Design review of the part built by this model. Coordinates are the model's own, in mm. Face numbers are marked on the shaded views. A direction names the side the tool comes from. Give positions to 0.01 mm unless a question says otherwise; leave off trailing zeros. Write each loop counter-clockwise with the first axis right and the second up, starting at its lowest first coordinate (ties: lowest second). Pieces come first, ordered by that corner, then holes. Notation, with made-up numbers: (3.5, -24) -> (23.5, -24) arc R20 cw to (23.5, -5) -> close; hole circle Ø1 at (-17, 16). An arc over 180 degrees is marked (long way). Use CSV: the item, a comma, the result in double quotes.
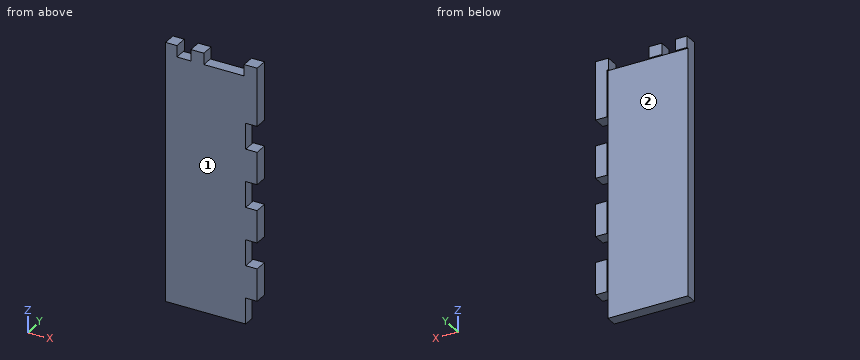
```python
from build123d import *

# Parameters (mm, degrees)
SKETCH1_W           = 44.958
SKETCH1_H           = 304.8
BOSS_EXTRUDE1_DEPTH = 5.588
SKETCH2_W           = 5.588
SKETCH2_H           = 101.6
BOSS_EXTRUDE2_DEPTH = 5.588
SKETCH3_W           = 121.412
SKETCH3_H           = 5.588
BOSS_EXTRUDE3_DEPTH = 39.37
SKETCH7_W           = 332.610738736
SKETCH7_H           = 323.725005723
CUT_EXTRUDE1_DEPTH  = 45.958
SKETCH4_W           = 5.588
SKETCH4_H           = 12.7
CUT_EXTRUDE2_DEPTH  = 6.35
SKETCH8_W           = 6.858
SKETCH8_H           = 5.588
SKETCH8_W_2         = 19.812
CUT_EXTRUDE4_DEPTH  = 7.35


with BuildPart() as part:
    # Sketch1 → Boss-Extrude1 (new body)
    with BuildSketch(Plane.XY):
        with Locations((-6.477, 3.048)):
            Rectangle(SKETCH1_W, SKETCH1_H)
        with BuildLine():
            Line((-3.302, 133.858), (-3.302, -143.002))
            Line((-3.302, -143.002), (3.302, -143.002))
            Line((3.302, -143.002), (3.302, 143.002))
            Line((3.302, 143.002), (-16.256, 143.002))
            Line((-16.256, 143.002), (-16.256, 136.398))
            Line((-16.256, 136.398), (-5.842, 136.398))
            ThreePointArc((-5.842, 136.398), (-4.045948776, 135.654051224), (-3.302, 133.858))
        make_face(mode=Mode.SUBTRACT)
    extrude(amount=BOSS_EXTRUDE1_DEPTH)

    # Sketch2 → Boss-Extrude2 (add)
    with BuildSketch(Plane(origin=(16.002, 0, 0), x_dir=(0, 0, -1), z_dir=(1, 0, 0))):
        Polygon((121.412, -60.452), (121.412, -47.752), (0, -47.752), (0, -149.352), (121.412, -149.352), (121.412, -136.652), (127, -136.652), (127, -119.718666667), (121.412, -119.718666667), (121.412, -107.018666667), (127, -107.018666667), (127, -90.085333333), (121.412, -90.085333333), (121.412, -77.385333333), (127, -77.385333333), (127, -60.452), align=None)
        with BuildLine():
            ThreePointArc((11.4, -116.592), (9.9, -118.092), (8.4, -116.592))
            Line((8.4, -116.592), (8.4, -111.512))
            ThreePointArc((8.4, -111.512), (9.9, -110.012), (11.4, -111.512))
            Line((11.4, -111.512), (11.4, -116.592))
        make_face(mode=Mode.SUBTRACT)
        with BuildLine():
            Line((42.4, -111.512), (42.4, -116.592))
            ThreePointArc((42.4, -116.592), (40.9, -118.092), (39.4, -116.592))
            Line((39.4, -116.592), (39.4, -111.512))
            ThreePointArc((39.4, -111.512), (40.9, -110.012), (42.4, -111.512))
        make_face(mode=Mode.SUBTRACT)
        with BuildLine():
            ThreePointArc((36.4, -101.092), (25.4, -112.092), (14.4, -101.092))
            Line((14.4, -101.092), (14.4, -96.012))
            ThreePointArc((14.4, -96.012), (25.4, -85.012), (36.4, -96.012))
            Line((36.4, -96.012), (36.4, -101.092))
        make_face(mode=Mode.SUBTRACT)
        with BuildLine():
            ThreePointArc((11.4, -85.592), (9.9, -87.092), (8.4, -85.592))
            Line((8.4, -85.592), (8.4, -80.512))
            ThreePointArc((8.4, -80.512), (9.9, -79.012), (11.4, -80.512))
            Line((11.4, -80.512), (11.4, -85.592))
        make_face(mode=Mode.SUBTRACT)
        with BuildLine():
            ThreePointArc((42.4, -85.592), (40.9, -87.092), (39.4, -85.592))
            Line((39.4, -85.592), (39.4, -80.512))
            ThreePointArc((39.4, -80.512), (40.9, -79.012), (42.4, -80.512))
            Line((42.4, -80.512), (42.4, -85.592))
        make_face(mode=Mode.SUBTRACT)
        with Locations((-2.794, -98.552)):
            Rectangle(SKETCH2_W, SKETCH2_H)
    extrude(amount=-BOSS_EXTRUDE2_DEPTH)

    # Sketch3 → Boss-Extrude3 (add)
    with BuildSketch(Plane.ZY.offset(-10.414)):
        with Locations((-60.706, -146.558)):
            Rectangle(SKETCH3_W, SKETCH3_H)
    extrude(amount=BOSS_EXTRUDE3_DEPTH)

    # Sketch7 → Cut-Extrude1 (cut, through all)
    with BuildSketch(Plane(origin=(16.002, 0, 0), x_dir=(0, 0, -1), z_dir=(1, 0, 0))):
        with Locations((160.717369368, 18.860502861)):
            Rectangle(SKETCH7_W, SKETCH7_H)
    extrude(amount=-CUT_EXTRUDE1_DEPTH, mode=Mode.SUBTRACT)

    # Sketch4 → Cut-Extrude2 (cut)
    with BuildSketch(Plane.XZ.offset(149.352)):
        with Locations((13.208, -29.337)):
            Rectangle(SKETCH4_W, SKETCH4_H)
        with Locations((13.208, -57.912)):
            Rectangle(SKETCH4_W, SKETCH4_H)
        with Locations((13.208, -86.487)):
            Rectangle(SKETCH4_W, SKETCH4_H)
        with Locations((13.208, -115.062)):
            Rectangle(SKETCH4_W, SKETCH4_H)
    extrude(amount=-CUT_EXTRUDE2_DEPTH, mode=Mode.SUBTRACT)

    # Sketch8 → Cut-Extrude4 (cut, through all)
    with BuildSketch(Plane.XZ.offset(149.352)):
        with Locations((-19.939, 2.794)):
            Rectangle(SKETCH8_W, SKETCH8_H)
        with Locations((-0.254, 2.794)):
            Rectangle(SKETCH8_W_2, SKETCH8_H)
    extrude(amount=-CUT_EXTRUDE4_DEPTH, mode=Mode.SUBTRACT)


solid = part.part
```
(1) Take a section at D-D (z = -8). Write out the cut boundary in (x, y).
Established:
outline,"(-28.96, -149.35) -> (16, -149.35) -> (16, -143) -> (10.41, -143) -> (10.41, -143.76) -> (-28.96, -143.76) -> close"
(2) For line 1 along Z through (x, y) = (11, -148.25); line 2 along X through (y, z) = (-147, -112); line 3 along Y through (x, z) = (-13.5, -67), list the stretches that pass through material, from the lowest coordinate up. Write a range as [from, to].
Established:
line 1,"z = [-108.71, -92.84], [-80.14, -64.26], [-51.56, -35.69], [-22.99, 5.59]"
line 2,"x = [-28.96, 10.41]"
line 3,"y = [-149.35, -143.76]"
(3) Take a section at B-B (x = -14.5). Write out the cut boundary in (y, z), then the cut area to 3 significant figures.
Established:
outline,"(-149.35, -121.41) -> (-143.76, -121.41) -> (-143.76, 0) -> (-143, 0) -> (-143, 5.59) -> (-149.35, 5.59) -> close"
area,"714 mm2"
(4) Clearance check with flat-ended pins moving along their axes: pin 1 (1.7 mm diameter, centred on y = -146, z = -55, fed in from +X); pin 2 (3 mm diameter, centred on x = 12.5, y = -145, fed in from -Z). State where each tip first meets the part, or that it passes through.
Established:
pin 1,"stops at x = 10.41"
pin 2,"stops at z = -108.71"
(5) Take a section at A-A (x = 12.5). Write out the cut boundary in (y, z).
Established:
outline,"(-149.35, -108.71) -> (-143, -108.71) -> (-143, -92.84) -> (-149.35, -92.84) -> close; (-149.35, -80.14) -> (-143, -80.14) -> (-143, -64.26) -> (-149.35, -64.26) -> close; (-149.35, -51.56) -> (-143, -51.56) -> (-143, -35.69) -> (-149.35, -35.69) -> close; (-149.35, -22.99) -> (-143, -22.99) -> (-143, 5.59) -> (-149.35, 5.59) -> close"
(6) Tool access review of the marked faces 1 and 2: name each direction out of +Z, -Z, +X, -X, +Y, -Y from which nothing blocks a thin tool from reaching the whole face with its end or side.
Established:
face 1,"+Z, -Z, +X, -X, -Y"
face 2,"-Z, -X, +Y"
(7) Take a section at C-C (y = -145.5). Write out the cut boundary in (x, z), then the cut area to 3 significant figures.
Established:
outline,"(-28.96, -121.41) -> (10.41, -121.41) -> (10.41, -108.71) -> (16, -108.71) -> (16, -92.84) -> (10.41, -92.84) -> (10.41, -80.14) -> (16, -80.14) -> (16, -64.26) -> (10.41, -64.26) -> (10.41, -51.56) -> (16, -51.56) -> (16, -35.69) -> (10.41, -35.69) -> (10.41, -22.99) -> (16, -22.99) -> (16, 5.59) -> (9.65, 5.59) -> (9.65, 0) -> (-10.16, 0) -> (-10.16, 5.59) -> (-16.51, 5.59) -> (-16.51, 0) -> (-23.37, 0) -> (-23.37, 5.59) -> (-28.96, 5.59) -> close"
area,"5,280 mm2"
